Could you check a few things on this model? Use its own coordinates, in mm. A direction names the side the tool comes from. Give positions to 0.01 mm unless a question says otherwise; leave off trailing zeros. Order: outer loops, then holes, each group sorted by start corner. A loop starts at its lowest first (then second) coordinate and runs counter-clockwise, first axis right, second up.
(1) Imagine slicing it at A-A, the plane x = 0. Write out the boundary of the cut face in (y, z).
(2) Will these pins go through, and if not, where does the flat tip stop? pin 1 (15.5 mm diameter, centred on x = -0.5, y = 11, fed in from +Z); pin 2 (1 mm diameter, centred on y = 2, z = 6.5, fed in from -X); pin 3 (4 mm diameter, centred on x = -13, z = 2, fed in from -Y).
(3) If we mould it in two halves opening along X, with no side actions, what happens to faces 1 (the cylindrical face through (-5.961, -26.846, 4.636)), 2 (the flat face through (5, 12, 6.2)), 3 (the flat face through (-11, -11, 0))? For each: released by +X, released by -X, zero draft, split by the parting line, or undercut.
(4) On a 3-axis mill with a long thin cutter (end or side, diameter ignored), from which of +Z, -Z, +X, -X, +Y, -Y can I reach the whole of each face in a straight line? I mean faces 4 (the cylindrical face through (-20.633, -15.821, 6.693)), 5 (the cylindrical face through (-2.764, -12.447, 3.564)). Say none if no direction works.
(5) If I drill on probe 1 along Y at (x, z) = (0, 6.5); probe 2 along Y at (x, z) = (0, 2.5); probe 3 along Z at (x, y) = (-7, 21), over which ranges is the centre line in solid material (lowest first)?
from build123d import *

# Parameters (mm, degrees)
F2_SIZE = 2
F3_SIZE = 1


with BuildPart() as f1:
    # F0 (on Front) → F1 (revolve)
    with BuildSketch(Plane.XZ):
        Polygon((12.75, 6.2), (12.75, 0), (27.5, 0), (27.5, 7.2), (26, 7.2), (26, 6.2), align=None)
    revolve(axis=Axis((0, 0, 15.391572), (0, 0, 1)))

    # F2
    f2_edges = [f1.edges().sort_by_distance(p)[0] for p in [
        (-27.5, 0, 0),
    ]]
    chamfer(f2_edges, length=F2_SIZE)

    # F3
    f3_edges = [f1.edges().sort_by_distance(p)[0] for p in [
        (-12.75, 0, 0),
    ]]
    chamfer(f3_edges, length=F3_SIZE)


solid = f1.part
Answer block:
1. outline: (-27.5, 2) - (-25.5, 0) - (-13.75, 0) - (-12.75, 1) - (-12.75, 6.2) - (-26, 6.2) - (-26, 7.2) - (-27.5, 7.2) - close; (12.75, 1) - (13.75, 0) - (25.5, 0) - (27.5, 2) - (27.5, 7.2) - (26, 7.2) - (26, 6.2) - (12.75, 6.2) - close
2. pin 1: stops at z = 6.2
2. pin 2: stops at x = -27.46
2. pin 3: stops at y = -25.2
3. face 1: split by the parting line
3. face 2: undercut
3. face 3: zero draft
4. face 4: +Z
4. face 5: +Z, -Z
5. probe 1: y = -27.5 to -26, 26 to 27.5
5. probe 2: y = -27.5 to -12.75, 12.75 to 27.5
5. probe 3: z = 0 to 6.2
